Autodesk Inventor part; units mm, degrees
ref_plane "YZ Plane" through (0, 0, 0) normal (1, 0, 0) x (0, 1, 0)
ref_plane "XZ Plane" through (0, 0, 0) normal (0, 1, 0) x (-1, 0, 0)
ref_plane "XY Plane" through (0, 0, 0) normal (0, 0, 1) x (1, 0, 0)
sketch "Sketch1" plane through (0, 0, 0) normal (0, 1, 0) x (-1, 0, 0)
  circle A0 centre (0, 0) radius 9.5
  circle A1 centre (0, 0) radius 2.4
  dimension "d0" = 19
  dimension "d1" = 4.8
extrude "Extrusion1" add sketch "Sketch1" along normal blind 3.18
sketch "Sketch2" plane through (0, 3.18, 0) normal (0, 1, 0) x (1, 0, 0)
  circle A0 centre (0, 0) radius 2.4
  circle A1 centre (0, 0) radius 4
  circle A2 centre (0, 0) radius 2.4
  dimension "d4" = 8
extrude "Extrusion2" add sketch "Sketch2" along normal blind 6.5
sketch "Sketch3" plane through (0, 3.18, 0) normal (0, 1, 0) x (1, 0, 0)
  circle A0 centre (-6.35, 0) radius 1.45
  circle A1 centre (0, 0) radius 6.35 construction
  dimension "d8" = 12.7
  dimension "d7" = 2.9
extrude "Extrusion3" cut sketch "Sketch3" against normal blind 6.5
pattern_circular "Circular Pattern1" count 3 over 360 about axis through (0, 3.18, 0) along (0, 1, 0) of "Extrusion3"
chamfer "Chamfer1" distance 0.5 angle 45 3 edges at (-4, 9.68, 0) (9.5, 3.18, 0) (9.5, 0, 0)
properties part number "Nut"
Input: part model. Units: mm. Frame: model coordinates. A direction names the side the tool comes from. Coordinates: 2 decimals unless noted, no trailing zeros. Loops run counter-clockwise (first coordinate to the right, second up) from the corner with the lowest first, then second, coordinate; pieces in that order, holes last. Notation, with made-up numbers: (78.25, 44.25) -> (108.25, 44.25) arc R24 ccw to (108.25, 58.25) -> close; hole circle Ø1 at (-29.5, -26). An arc over 180 degrees is marked (long way). Write each question's results on one line, items separated by ' | '. Start each with the question number.
Q1. Reachability of faces 1 (the cylindrical face through (0.158, 4.772, 2.395)), 2 (the flat face through (-4, 3.18, -2)) from +Z, -Z, +X, -X, +Y, -Y: full face, straight path, thin tool, end or side. Return the list, or none.
Q2. Ray query, line 1 (Z direction, x = 0, y = 5); line 2 (Y direction, x = -4.75, z = 2.25); line 3 (Z direction, x = -0.5, y = 6.5). Return the intervals inside material, ascending. Write a range as from..to.
Q3. Pin query (flat end, axial travel): pin 1 (5 mm diameter, centred on x = 0, y = 6.5, fed in from +Z); pin 2 (4.5 mm diameter, centred on x = -6.35, z = 0, fed in from +Y); pin 3 (4 mm diameter, centred on x = -4, y = 7, fed in from -Z). Return the tip coordinate at first contact, or that it passes through.
Q4. Section C-C, the plane x = 3.25. State how many separate pieces and enclosed holes the cut face has, plus the area to 3 significant figures.
Q5. Section B-B, the plane y = 2. Return the cut outline in (x, z) (3 decimals).
Q6. Pull-direction query (Z, two-part tool) for faces 3 (the cylindrical face through (-0.867, 6.138, -3.905)), 4 (the cylindrical face through (2.99, 1.61, 4.06)), 5 (the flat face through (-2, 0, -2)); classes: released by +Z, released by -Z, zero draft, split by the parting line, or undercut.
Found:
1) face 1: +Y, -Y | face 2: +Y
2) line 1: -4..-2.4, 2.4..4 | line 2: 0..3.18 | line 3: -3.97..-2.35, 2.35..3.97
3) pin 1: z = 4 | pin 2: y = 3.18 | pin 3: z = -3.46
4) separate pieces: 3 | enclosed holes: 0 | area: 67.7 mm2
5) outline: circle Ø19 at (0, 0); hole circle Ø2.9 at (-6.35, 0); hole circle Ø4.8 at (0, 0); hole circle Ø2.9 at (3.175, -5.499); hole circle Ø2.9 at (3.175, 5.499)
6) face 3: split by the parting line | face 4: undercut | face 5: zero draft
